Input: part model. Units: mm. Frame: model coordinates. Face numbers are marked on the shaded views. A direction names the side the tool comes from. Give positions to 0.01 mm unless a question says otherwise; leave off trailing zeros. Loops run counter-clockwise (first coordinate to the right, second up) from the corner with the lowest first, then second, coordinate; pieces in that order, holes last. Notation, with made-up numbers: (40, 24.5) -> (61, 24.5) arc R12 ccw to (61, 43.5) -> close; hole circle Ø10 at (58, 52.25). An arc over 180 degrees is marked (long way). Answer in a Markdown table with one row per item. Add a question column.
```python
from build123d import *

# Parameters (mm, degrees)
SKETCH_1_R          = 18.5
EXTRUDE_1_DEPTH     = 27
SKETCH_2_R          = 17.5
EXTRUDE_2_DEPTH     = 30
SKETCH_3_R          = 2.75
CUT_EXTRUDE_1_DEPTH = 24.4
SKETCH_4_R          = 1.6
SKETCH_4_R_2        = 2.75
CUT_EXTRUDE_2_DEPTH = 10


with BuildPart() as part:
    # 草图1 → 凸台-拉伸1 (new body)
    with BuildSketch(Plane.XY):
        Circle(SKETCH_1_R)
    extrude(amount=EXTRUDE_1_DEPTH)

    # 草图2 → 凸台-拉伸2 (add)
    with BuildSketch(Plane.XY.offset(27)):
        Circle(SKETCH_2_R)
    extrude(amount=EXTRUDE_2_DEPTH)

    # 草图3 → 切除-拉伸1 (cut)
    with BuildSketch(Plane(origin=(0, 0, 0), x_dir=(-1, 0, 0), z_dir=(0, 0, -1))):
        with Locations((0, -9.25)):
            Circle(SKETCH_3_R)
    extrude(amount=-CUT_EXTRUDE_1_DEPTH, mode=Mode.SUBTRACT)

    # 草图4 → 切除-拉伸2 (cut)
    with BuildSketch(Plane(origin=(0, 0, 0), x_dir=(-1, 0, 0), z_dir=(0, 0, -1))):
        with Locations((-16, -1.25)):
            Circle(SKETCH_4_R)
        with Locations((-8, 11.75)):
            Circle(SKETCH_4_R)
        with Locations((0, -9.25)):
            Circle(SKETCH_4_R_2)
        with Locations(Location((16, -1.25, 0), (0, 0, 180))):
            Circle(SKETCH_4_R)
        with Locations(Location((8, 11.75, 0), (0, 0, 180))):
            Circle(SKETCH_4_R)
    extrude(amount=-CUT_EXTRUDE_2_DEPTH, mode=Mode.SUBTRACT)


solid = part.part
```
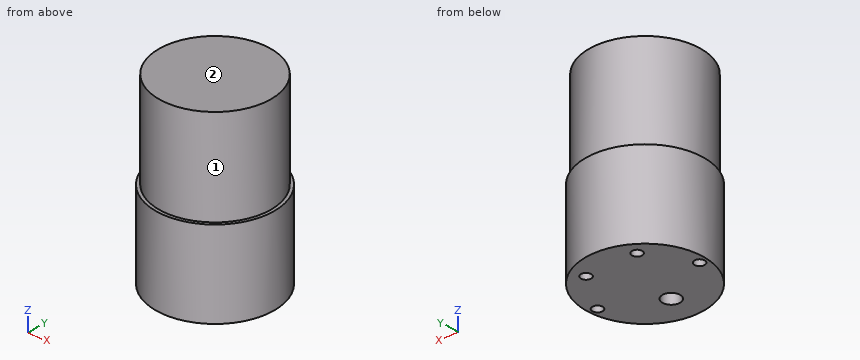
1) Section B-B on z = 12.5. Output: boundary loops of the cut face in (x, y), and give its area (3 significant figures).
2) Pin query (flat end, axial travel): pin 1 (1 mm diameter, centred on x = -7.5, y = 11.5, fed in from -Z); pin 2 (10 mm diameter, centred on y = -10, z = 9, fed in from -X); pin 3 (1 mm diameter, centred on y = 1.5, z = 37, fed in from -X). Return the tip coordinate at first contact, or that it passes through.
3) Reachability of the marked faces 1 and 2 from +Z, -Z, +X, -X, +Y, -Y: full face, straight path, thin tool, end or side. Return the list, or none.
4) Section C-C on y = -9.25. Output: boundary loops of the cut face in (x, z).
5) Section D-D on z = 45. Output: boundary loops of the cut face in (x, y).
6) Material intervals for line 1 along X through (y, z) = (11, 8); line 2 along X through (y, z) = (-0.5, 32.5); line 3 along Z through (x, y) = (-12.5, -12.5), sorted ascending.
7) Section A-A on x = 0. Output: boundary loops of the cut face in (y, z), and give its area (3 significant figures).
Working result:
| question | item | result |
|---|---|---|
| 1 | outline | circle Ø37 at (0, 0); hole circle Ø5.5 at (0, -9.25) |
| 1 | area | 1,050 mm2 |
| 2 | pin 1 | stops at z = 10 |
| 2 | pin 2 | stops at x = -17.81 |
| 2 | pin 3 | stops at x = -17.47 |
| 3 | face 1 | +Z |
| 3 | face 2 | +Z, +X, -X, +Y, -Y |
| 4 | outline | (-16.02, 0) -> (-2.75, 0) -> (-2.75, 24.4) -> (2.75, 24.4) -> (2.75, 0) -> (16.02, 0) -> (16.02, 27) -> (14.86, 27) -> (14.86, 57) -> (-14.86, 57) -> (-14.86, 27) -> (-16.02, 27) -> close |
| 5 | outline | circle Ø35 at (0, 0) |
| 6 | line 1 | x = -14.87 to -9.41, -6.59 to 6.59, 9.41 to 14.87 |
| 6 | line 2 | x = -17.49 to 17.49 |
| 6 | line 3 | z = 0 to 27 |
| 7 | outline | (-18.5, 0) -> (-12, 0) -> (-12, 24.4) -> (-6.5, 24.4) -> (-6.5, 0) -> (18.5, 0) -> (18.5, 27) -> (17.5, 27) -> (17.5, 57) -> (-17.5, 57) -> (-17.5, 27) -> (-18.5, 27) -> close |
| 7 | area | 1,910 mm2 |
